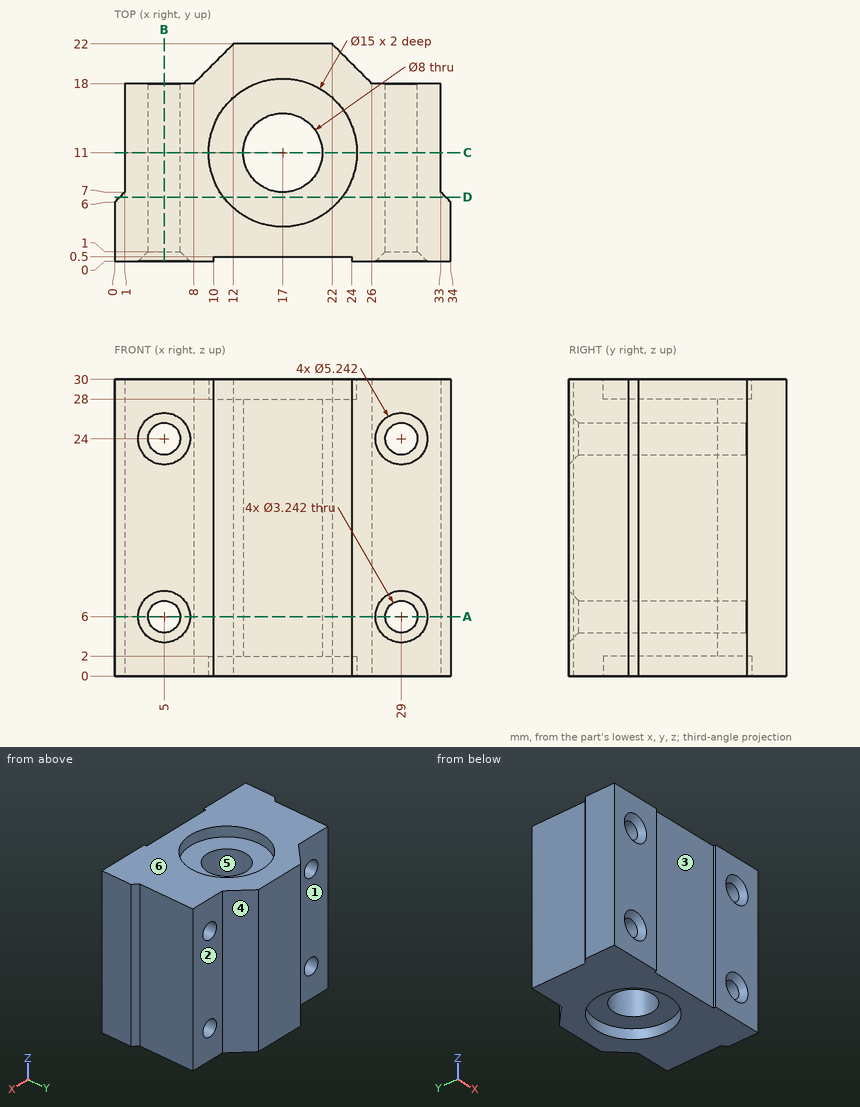
Drawing for the job (mm, zero at the part's lowest x, y, z). A direction names the side the tool comes from. Round coordinates to 2 decimals unless told otherwise and drop trailing zeros. Write each loop counter-clockwise with the first axis right and the second up, starting at its lowest first coordinate (ties: lowest second). Pieces come first, ordered by that corner, then holes. Notation, with made-up numbers: (58.5, 35) - (106.5, 35) arc R28 cw to (106.5, 67) - close; hole circle Ø7 at (16.5, 35.25). An arc over 180 degrees is marked (long way). Return JSON: item names as keys, results as strings. Group by question number.
Item 1: Band-saw the part on B-B on x = 5. List the corners of the cut face in (y, z).
Item 2: Band-saw the part on D-D on y = 6.5. List the corners of the cut face in (x, z), plus the area to 3 significant figures.
Item 3: Band-saw the part on C-C on y = 11. List the corners of the cut face in (x, z), plus the area to 3 significant figures.
Item 4: Probe probe 1 along Z at (x, y) = (29, 13); probe 2 along X at (y, z) = (14, 6); probe 3 along Y at (x, z) = (17, 1.6). List the from-to ranges inside material, lowest first.
Item 5: Band-saw the part on A-A on z = 6. State how many separate pieces and enclosed holes the cut face has, plus the area to 3 significant figures.
Item 6: Mould opens along Y. For the marked faces 4, 5 and 6 say: +Y half, -Y half, draft (parallel to the pull), parting line (faces both ways), or undercut.
Item 7: 3-axis set-ups, long thin cutter, end or side, ignore diameter. For the marked faces 1, 2 and 3: which of +Z, -Z, +X, -X, +Y, -Y reach the whole face in a straight line?
Item 8: Flat gauge pins, fed straight in: pin 1 Ø12 at (x, y) = (17, 11) entering from +Z; pin 2 Ø5 at (x, z) = (29, 6) entering from -Y; pin 3 Ø2 at (x, z) = (3, 16.5) entering from +Y. Where does each tip first touch, or does it go through?
Resolved:
{
 "1": {"outline": "(0, 0) - (18, 0) - (18, 4.38) - (1, 4.38) - (0, 3.38) - close; (0, 8.62) - (1, 7.62) - (18, 7.62) - (18, 22.38) - (1, 22.38) - (0, 21.38) - close; (0, 26.62) - (1, 25.62) - (18, 25.62) - (18, 30) - (0, 30) - close"},
 "2": {"outline": "(0.5, 0) - (11, 0) - (11, 2) - (23, 2) - (23, 0) - (33.5, 0) - (33.5, 30) - (23, 30) - (23, 28) - (11, 28) - (11, 30) - (0.5, 30) - close; hole circle Ø3.24 at (5, 6); hole circle Ø3.24 at (5, 24); hole circle Ø3.24 at (29, 6); hole circle Ø3.24 at (29, 24)", "area": "909 mm²"},
 "3": {"outline": "(1, 0) - (9.5, 0) - (9.5, 2) - (13, 2) - (13, 28) - (9.5, 28) - (9.5, 30) - (1, 30) - close; (21, 2) - (24.5, 2) - (24.5, 0) - (33, 0) - (33, 30) - (24.5, 30) - (24.5, 28) - (21, 28) - close; hole circle Ø3.24 at (5, 6); hole circle Ø3.24 at (5, 24); hole circle Ø3.24 at (29, 6); hole circle Ø3.24 at (29, 24)", "area": "659 mm²"},
 "4": {"probe 1": "z = 0 to 4.38, 7.62 to 22.38, 25.62 to 30", "probe 2": "x = 1 to 3.38, 6.62 to 14.35, 19.65 to 27.38, 30.62 to 33", "probe 3": "y = 0.5 to 3.5, 18.5 to 22"},
 "5": {"separate pieces": "3", "enclosed holes": "1", "area": "469 mm²"},
 "6": {"face 4": "+Y half", "face 5": "undercut", "face 6": "draft"},
 "7": {"face 1": "+Z, -Z, -X, +Y", "face 2": "+Z, -Z, +X, +Y", "face 3": "+Z, -Z, -Y"},
 "8": {"pin 1": "stops at z = 28", "pin 2": "stops at y = 0.12", "pin 3": "stops at y = 18"}
}
